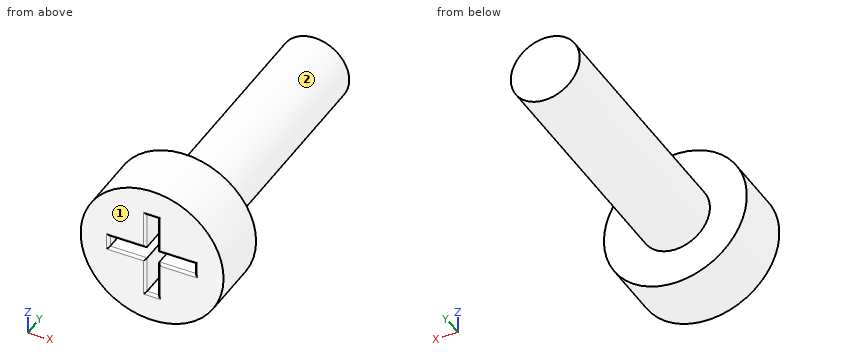
```python
from build123d import *

# Parameters (mm, degrees)
F0_R     = 1.4
F1_DEPTH = 10
F3_R     = 2.9
F4_DEPTH = 2.5
F3_W     = 0.5
F3_H     = 0.5
F3_W_2   = 1.5
F3_H_2   = 1.5
F5_DEPTH = 0.5
F6_R     = 0.1


with BuildPart() as f1:
    # F0 (on Front) → F1 (new body)
    with BuildSketch(Plane.XZ):
        Circle(F0_R)
    extrude(amount=F1_DEPTH)

    # F3 (on offset) → F4 (join)
    with BuildSketch(Plane.XZ.offset(10)):
        Circle(F3_R)
        Polygon((0.25, -0.25), (0.25, -1.75), (-0.25, -1.75), (-0.25, -0.25), (-1.75, -0.25), (-1.75, 0.25), (-0.25, 0.25), (-0.25, 1.75), (0.25, 1.75), (0.25, 0.25), (1.75, 0.25), (1.75, -0.25), align=None, mode=Mode.SUBTRACT)
    extrude(amount=F4_DEPTH)

    # F3 (on offset) → F5 (join)
    with BuildSketch(Plane.XZ.offset(10)):
        Rectangle(F3_W, F3_H)
        with Locations((-1, 0)):
            Rectangle(F3_W_2, F3_H)
        with Locations((0, -1)):
            Rectangle(F3_W, F3_H_2)
        with Locations((1, 0)):
            Rectangle(F3_W_2, F3_H)
        with Locations((0, 1)):
            Rectangle(F3_W, F3_H_2)
    extrude(amount=F5_DEPTH)

    # F6
    f6_edges = [f1.edges().sort_by_distance(p)[0] for p in [
        (-0.25, -12.5, 1),
        (-1, -12.5, 0.25),
        (-1, -12.5, -0.25),
        (-0.25, -12.5, -1),
        (-1.75, -12.5, 0),
        (0.25, -12.5, -1),
        (0, -12.5, -1.75),
        (1, -12.5, -0.25),
        (1.75, -12.5, 0),
        (0.25, -12.5, 1),
        (0, -12.5, 1.75),
        (1, -12.5, 0.25),
    ]]
    fillet(f6_edges, radius=F6_R)


solid = f1.part
```
Read the model definition and answer for the solid it produces. Units are mm, in the model's axes. Face numbers are marked on the shaded views. A direction names the side the tool comes from. Coordinates: 2 decimals unless noted, no trailing zeros. Loops run counter-clockwise (first coordinate to the right, second up) from the corner with the lowest first, then second, coordinate; pieces in that order, holes last. Notation, with made-up numbers: (-12.5, 39.25) - (21.5, 39.25) arc R19 cw to (21.5, 68.25) - close; hole circle Ø10 at (88.25, -32.75). An arc over 180 degrees is marked (long way). Answer in a Markdown table with one row per item.
1. Find section B-B, the plane x = 0. Write down the section's boundary in (y, z), then the cut area to 3 significant figures.
Conclusion:
| item | result |
|---|---|
| outline | (-12.5, -2.9) - (-10, -2.9) - (-10, -1.4) - (0, -1.4) - (0, 1.4) - (-10, 1.4) - (-10, 2.9) - (-12.5, 2.9) - (-12.5, 1.85) arc R0.1 ccw to (-12.4, 1.75) - (-10.5, 1.75) - (-10.5, -1.75) - (-12.4, -1.75) arc R0.1 ccw to (-12.5, -1.85) - close |
| area | 35.5 mm² |
2. Which of the six approach directions +Z, -Z, +X, -X, +Y, -Y give full straight-line access (tool end or side, diameter ignored) to the marked faces 1 and 2?
Conclusion:
| item | result |
|---|---|
| face 1 | +Z, -Z, +X, -X, -Y |
| face 2 | +Y |
3. Find section A-A, the plane y = -11.5. Write down the section's boundary in (x, z), then the cut area to 3 significant figures.
Conclusion:
| item | result |
|---|---|
| outline | circle Ø5.8 at (0, 0); hole (-1.75, -0.25) - (-0.25, -0.25) - (-0.25, -1.75) - (0.25, -1.75) - (0.25, -0.25) - (1.75, -0.25) - (1.75, 0.25) - (0.25, 0.25) - (0.25, 1.75) - (-0.25, 1.75) - (-0.25, 0.25) - (-1.75, 0.25) - close |
| area | 23.2 mm² |
4. Given pin 1 (1.5 mm diameter, centred on x = 0, y = -8.5, fed in from -Z); pin 2 (1.6 mm diameter, centred on x = 1, y = -11.5, fed in from -Z); pin 3 (1.2 mm diameter, centred on y = -11, z = 1, fed in from -X); pin 4 (1.7 mm diameter, centred on x = 0.5, z = -0.5, fed in from +Y), each flat-ended and moving along its own axis, determine where each tip first touches the part or whether it passes through.
Conclusion:
| item | result |
|---|---|
| pin 1 | stops at z = -1.4 |
| pin 2 | stops at z = -2.89 |
| pin 3 | stops at x = -2.87 |
| pin 4 | stops at y = 0 |
5. Straight lines are drawn through the part: line 1 (Y direction, x = -0.25, z = -2); line 2 (Y direction, x = -0.15, z = 0.7); line 3 (X direction, y = -11, z = -0.85). For each, find the intervals that lie inside material, in ascending order.
Conclusion:
| item | result |
|---|---|
| line 1 | y = -12.5 to -10 |
| line 2 | y = -10.5 to 0 |
| line 3 | x = -2.77 to -0.25, 0.25 to 2.77 |
6. Find section C-C, the plane z = 0. Write down the section's boundary in (x, y).
Conclusion:
| item | result |
|---|---|
| outline | (-2.9, -12.5) - (-1.85, -12.5) arc R0.1 ccw to (-1.75, -12.4) - (-1.75, -10.5) - (1.75, -10.5) - (1.75, -12.4) arc R0.1 ccw to (1.85, -12.5) - (2.9, -12.5) - (2.9, -10) - (1.4, -10) - (1.4, 0) - (-1.4, 0) - (-1.4, -10) - (-2.9, -10) - close |
7. Find section D-D, the plane y = -6.5. Write down the section's boundary in (x, z).
Conclusion:
| item | result |
|---|---|
| outline | circle Ø2.8 at (0, 0) |
